Could you check a few things on this drawing? It's one solid part, dimensions in mm from its lowest x, y, z. Coordinates: 2 decimals unless noted, no trailing zeros. Write each loop counter-clockwise with the first axis right and the second up, starting at its lowest first coordinate (ties: lowest second). Pieces come first, ordered by that corner, then holes. Notation, with made-up numbers: (42.5, 75.5) - (100.5, 75.5) arc R19 cw to (100.5, 83.5) - close; hole circle Ø4 at (19, -10). An arc over 180 degrees is marked (long way). Use one line per item in the form item = value. Start each with the question number.
(1) If I drill on probe 1 along X at (y, z) = (2, 0.8); probe 2 along Y at (x, z) = (222, 3.4); probe 3 along X at (y, z) = (27.5, 1.4), over which ranges is the centre line in solid material (lowest first)? Write a range as from..to.
(2) Thinking about a two-plate mould opening in Z: for the marked faces 1 and 2, which applies, pulls with the +Z half, pulls with the -Z half, needs draft (parallel to the pull), parting line crosses it, or undercut?
(3) For pin 1 Ø2 at (x, z) = (370.5, 2) entering from +Y; pin 2 Ø2 at (y, z) = (2.5, 2.5) entering from -X; pin 3 Ø2 at (x, z) = (65.5, 1) entering from -Y, each with a flat end and sliding along its axis, tell me the tip position at first contact or that it passes through.
(4) If we section it at A-A on x = 155: Please give me the cut outline in (y, z).
(5) If we section it at B-B on y = 25: Please give me the cut outline in (x, z).
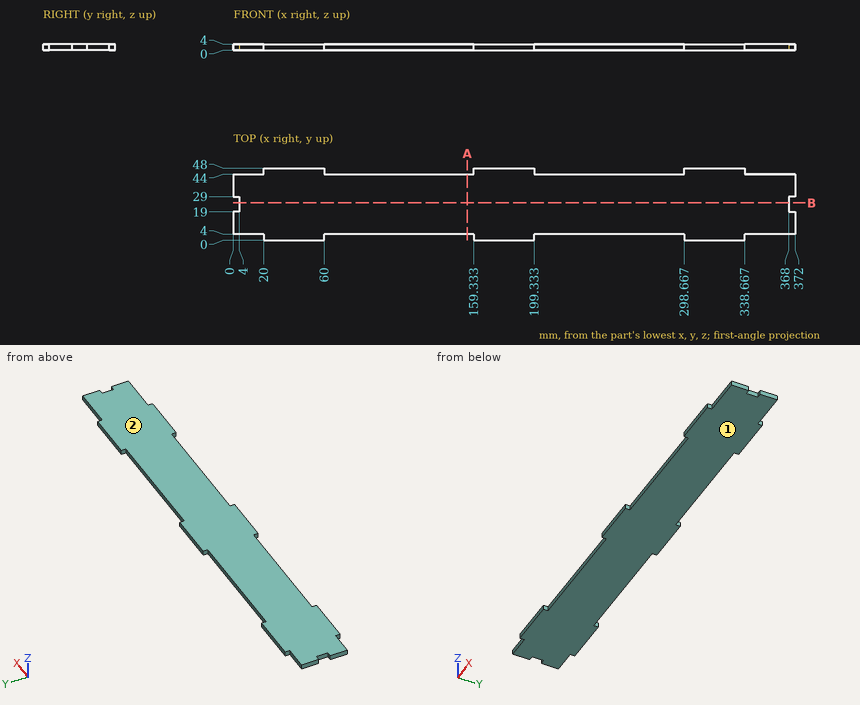
Reported:
q1.probe_1 = 20..60, 159.33..199.33, 298.67..338.67
q1.probe_2 = 4..44
q1.probe_3 = 4..368
q2.face_1 = pulls with the -Z half
q2.face_2 = pulls with the +Z half
q3.pin_1 = 44
q3.pin_2 = 20
q3.pin_3 = 4
q4.outline = (4, 0) - (44, 0) - (44, 4) - (4, 4) - close
q5.outline = (4, 0) - (368, 0) - (368, 4) - (4, 4) - close
